CAD build for the part. Positions are in the model's coordinates, mm. A direction names the side the tool comes from. Coordinates: 2 decimals unless noted, no trailing zeros. Order: outer loops, then holes, each group sorted by start corner. A loop starts at its lowest first (then second) coordinate and runs counter-clockwise, first axis right, second up. Notation, with made-up numbers: M 76,-35 L 105,-35 A27 cw 105,-12 Z; hole C 50,21.5 d3. An arc over 180 degrees is marked long. Write item = value, one per line.
from build123d import *

# Parameters (mm, degrees)
F1_DEPTH = 850


with BuildPart() as f1:
    # F0 (on Front) → F1 (new body, symmetric)
    with BuildSketch(Plane.XZ):
        with BuildLine():
            ThreePointArc((25, 23), (24.414214, 24.414214), (23, 25))
            Line((23, 25), (-23, 25))
            ThreePointArc((-23, 25), (-24.414214, 24.414214), (-25, 23))
            Line((-25, 23), (-25, -23))
            ThreePointArc((-25, -23), (-24.414214, -24.414214), (-23, -25))
            Line((-23, -25), (23, -25))
            ThreePointArc((23, -25), (24.414214, -24.414214), (25, -23))
            Line((25, -23), (25, 23))
        make_face()
        with BuildLine():
            Line((-20.5, 22.5), (20.5, 22.5))
            ThreePointArc((20.5, 22.5), (21.914214, 21.914214), (22.5, 20.5))
            Line((22.5, 20.5), (22.5, -20.5))
            ThreePointArc((22.5, -20.5), (21.914214, -21.914214), (20.5, -22.5))
            Line((20.5, -22.5), (-20.5, -22.5))
            ThreePointArc((-20.5, -22.5), (-21.914214, -21.914214), (-22.5, -20.5))
            Line((-22.5, -20.5), (-22.5, 20.5))
            ThreePointArc((-22.5, 20.5), (-21.914214, 21.914214), (-20.5, 22.5))
        make_face(mode=Mode.SUBTRACT)
    extrude(amount=F1_DEPTH, both=True)


solid = f1.part
(1) Slice it at C-C, the plane y = 352. Write the cut outline in (x, z).
Evaluation:
outline = M -25,-23 A2 ccw -23,-25 L 23,-25 A2 ccw 25,-23 L 25,23 A2 ccw 23,25 L -23,25 A2 ccw -25,23 Z; hole M -22.5,-20.5 A2 ccw -20.5,-22.5 L 20.5,-22.5 A2 ccw 22.5,-20.5 L 22.5,20.5 A2 ccw 20.5,22.5 L -20.5,22.5 A2 ccw -22.5,20.5 Z
(2) Tool access for faces 1 (the face through (0, -12, -25)), 2 (the face through (-22.5, -12, 0)): list every direction of +Z, -Z, +X, -X, +Y, -Y with a clear straight run to the whole face (end or side of a thin tool).
Evaluation:
face_1 = -Z, +X, -X, +Y, -Y
face_2 = +Y, -Y
(3) Pull direction Z, two halves, no side cores. Call faces 3 (the face through (25, -12, 0)), 4 (the face through (0, -12, 25)), 5 (the face through (0, -12, 22.5)): +Z half, -Z half, draft (parallel to the pull), parting line (faces both ways), or undercut.
Evaluation:
face_3 = draft
face_4 = +Z half
face_5 = undercut
(4) Slice it at A-A, the plane z = 3.5. Write the cut outline in (x, y), then the cut area to 3 significant figures.
Evaluation:
outline = M -25,-850 L -22.5,-850 L -22.5,850 L -25,850 Z; M 22.5,-850 L 25,-850 L 25,850 L 22.5,850 Z
area = 8,500 mm²
(5) Slice it at B-B, the plane x = -11. Write the cut outline in (y, z).
Evaluation:
outline = M -850,-25 L 850,-25 L 850,-22.5 L -850,-22.5 Z; M -850,22.5 L 850,22.5 L 850,25 L -850,25 Z
(6) Wall check: line 1 (Z direction, x = -6.5, y = -309); line 2 (X direction, y = -552, z = -21). Give the ranges that are in metal, low to high. Write a range as from..to.
Evaluation:
line_1 = -25..-22.5, 22.5..25
line_2 = -25..-22.44, 22.44..25
(7) Pin check, flat tip, straight feed: pin 1 Ø3 at (x, z) = (-19.5, 9.5) entering from +Y. Stop position of the tip, or through.
Evaluation:
pin_1 = through
